Design review of the part built by this model. Coordinates are the model's own, in mm. Face numbers are marked on the shaded views. A direction names the side the tool comes from. Round coordinates to 2 decimals unless told otherwise and drop trailing zeros. Order: outer loops, then holes, each group sorted by start corner. A loop starts at its lowest first (then second) coordinate and runs counter-clockwise, first axis right, second up. Notation, with made-up numbers: M 23.25,31 L 35.25,31 A15 cw 35.25,55 Z; hole C 60,20 d2. An arc over 180 degrees is marked long. Use a Markdown table: item, result. Add a question column.
(1) Take a section at A-A (y = -15). Write out the cut boundary in (x, z), then the cut area to 3 significant figures.
(2) Machinability: for the marked faces 4 and 5, which of the approach directions +Z, -Z, +X, -X, +Y, -Y give a long, thin tool a straight path to every point of the face, cutting with its end or side? Answer none if there is none.
(3) To check wall thickness, follow probe 1 along Y at (x, z) = (-4, -3.5); probe 2 along Z at (x, y) = (0, -24); probe 3 along X at (y, z) = (8, 0). State the ranges of each line that lie inside material, in increasing order. Write a range as from..to.
(4) Take a section at C-C (z = -5.25). Write out the cut boundary in (x, y), then the cut area to 3 significant figures.
(5) For pin 1 (0.8 mm diameter, centred on y = 17, z = -2, fed in from +X); pin 2 (12 mm diameter, centred on x = -3.5, y = 11, fed in from +Z); pin 3 (1.8 mm diameter, centred on x = 0, z = 0, fed in from -Y); pin 4 (6 mm diameter, centred on y = 12, z = 2, fed in from +X), all flat-tipped, find the tip position at first contact; note any pin that passes through.
(6) The part is to be moulded in two halves that separate along X. For the marked faces 1, 2 and 3, say which applies: released by +X, released by -X, zero draft, split by the parting line, or undercut.
(7) Take a section at D-D (z = 0). Count the separate pieces of the cut face and the enclosed holes in it, then the cut area to 3 significant figures.
(8) Take a section at B-B (x = 14). Write out the cut boundary in (y, z), then the cut area to 3 significant figures.
```python
from build123d import *

# Parameters (mm, degrees)
F1_W     = 1
F1_H     = 12
F3_R     = 1
F4_DEPTH = 1
F5_R     = 1
F6_DEPTH = 1
F7_R     = 1
F8_DEPTH = 1


with BuildPart() as f2:
    # F2: sweep along a path in F0
    with BuildLine(Plane.XY) as f2_path:
        Line((0, 17.3205080757), (0.268994947, 17.3205080757))
        Line((0.268994947, 17.3205080757), (16.8452994616, 17.3205080757))
        ThreePointArc((16.8452994616, 17.3205080757), (17.8461933486, 17.0520424897), (18.5783816717, 16.3187195027))
        Line((18.5783816717, 16.3187195027), (23.4179019593, 7.9164048343))
        ThreePointArc((23.4179019593, 7.9164048343), (23.6848194828, 6.9171610817), (23.4168705568, 5.9181934072))
        Line((23.4168705568, 5.9181934072), (6.5773502692, -23.248711306))
        ThreePointArc((6.5773502692, -23.248711306), (5.8452994616, -23.9807621135), (4.8452994616, -24.248711306))
        Line((4.8452994616, -24.248711306), (-4.8452994616, -24.248711306))
        ThreePointArc((-4.8452994616, -24.248711306), (-5.8452994616, -23.9807621135), (-6.5773502692, -23.248711306))
        Line((-6.5773502692, -23.248711306), (-23.4226497308, 5.9282032303))
        ThreePointArc((-23.4226497308, 5.9282032303), (-23.6905989232, 6.9282032303), (-23.4226497308, 7.9282032303))
        Line((-23.4226497308, 7.9282032303), (-18.5773502692, 16.3205080757))
        ThreePointArc((-18.5773502692, 16.3205080757), (-17.8452994616, 17.0525588833), (-16.8452994616, 17.3205080757))
        Line((-16.8452994616, 17.3205080757), (-0.3151426208, 17.3205080757))
    # F1 (on Right) → F2 (sweep)
    with BuildSketch(Plane.YZ):
        with Locations((17.3205080757, 0)):
            Rectangle(F1_W, F1_H)
    sweep(path=f2_path.line)

    # F3 (on face) → F4 (cut, through all)
    with BuildSketch(Plane.XZ.offset(24.748711306)):
        Circle(F3_R)
    extrude(amount=-F4_DEPTH, mode=Mode.SUBTRACT)

    # F5 (on face) → F6 (cut, through all)
    with BuildSketch(Plane(origin=(21.441430996, 12.3497208085, 0), x_dir=(-0.4991057135, 0.866541105, 0), z_dir=(0.866541105, 0.4991057135, 0))):
        Circle(F5_R)
    extrude(amount=-F6_DEPTH, mode=Mode.SUBTRACT)

    # F7 (on face) → F8 (cut, through all)
    with BuildSketch(Plane(origin=(-21.4330127019, 12.374355653, 0), x_dir=(-0.5, -0.8660254038, 0), z_dir=(-0.8660254038, 0.5, 0))):
        Circle(F7_R)
    extrude(amount=-F8_DEPTH, mode=Mode.SUBTRACT)


solid = f2.part
```
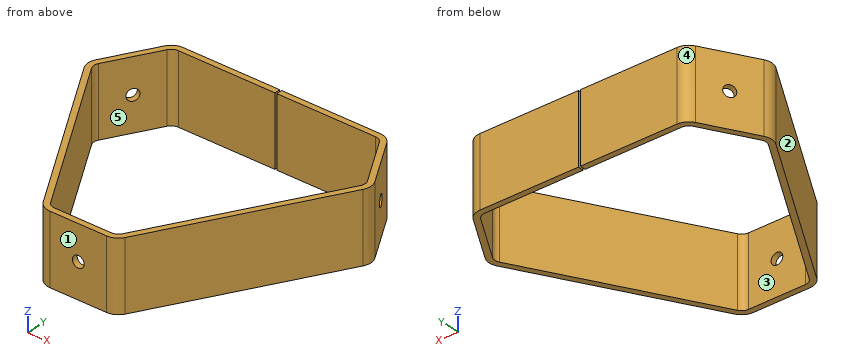
Verdict:
| question | item | result |
|---|---|---|
| 1 | outline | M -11.92,-6 L -10.76,-6 L -10.76,6 L -11.92,6 Z; M 10.76,-6 L 11.92,-6 L 11.92,6 L 10.76,6 Z |
| 1 | area | 27.7 mm^2 |
| 2 | face 4 | +Z, -Z, -X, +Y |
| 2 | face 5 | +Z, -Z |
| 3 | probe 1 | y = -24.75..-23.75, 16.82..17.82 |
| 3 | probe 2 | z = -6..-1, 1..6 |
| 3 | probe 3 | x = -23.95..-22.8, 22.79..23.94 |
| 4 | outline | M -23.86,5.68 L -7.01,-23.5 A2.5 ccw -4.85,-24.75 L 4.85,-24.75 A2.5 ccw 7.01,-23.5 L 23.85,5.67 A2.5 ccw 23.85,8.17 L 19.01,16.57 A2.5 ccw 16.85,17.82 L 0,17.82 L 0,16.82 L 16.85,16.82 A1.5 cw 18.15,16.07 L 22.98,7.67 A1.5 cw 22.98,6.17 L 6.14,-23 A1.5 cw 4.85,-23.75 L -4.85,-23.75 A1.5 cw -6.14,-23 L -22.99,6.18 A1.5 cw -22.99,7.68 L -18.14,16.07 A1.5 cw -16.85,16.82 L -0.32,16.82 L -0.32,17.82 L -16.85,17.82 A2.5 ccw -19.01,16.57 L -23.86,8.18 A2.5 ccw Z |
| 4 | area | 142 mm^2 |
| 5 | pin 1 | stops at x = 18.99 |
| 5 | pin 2 | stops at z = 6 |
| 5 | pin 3 | stops at y = 16.82 |
| 5 | pin 4 | stops at x = 23.37 |
| 6 | face 1 | zero draft |
| 6 | face 2 | released by -X |
| 6 | face 3 | undercut |
| 7 | separate pieces | 4 |
| 7 | enclosed holes | 0 |
| 7 | area | 136 mm^2 |
| 8 | outline | M -11.39,-6 L -9.39,-6 L -9.39,6 L -11.39,6 Z; M 16.82,-6 L 17.82,-6 L 17.82,6 L 16.82,6 Z |
| 8 | area | 36.0 mm^2 |
